Verification items for the finished model (mm, model axes). Coordinates: 2 decimals unless noted, no trailing zeros. Order: outer loops, then holes, each group sorted by start corner. A loop starts at its lowest first (then second) coordinate and runs counter-clockwise, first axis right, second up. Notation, with made-up numbers: (81.5, -21.5) -> (96.5, -21.5) arc R14 cw to (96.5, -1.5) -> close; hole circle Ø4 at (59, -12). An arc over 180 degrees is marked (long way). Use CSV: the item, a comma, the result in double quotes. Start each with the question number.
1) Release check for a two-part mould opening along X. For faces 1 (the flat face through (5.107, 38.792, 0.032)), 2 (the flat face through (-35, 10, 2.306)), 3 (the cylindrical face through (-42.5, 2.8, 0)) record: released by +X, released by -X, zero draft, split by the parting line, or undercut.
2) Go/stop test with flat-tipped pins: pin 1 (8 mm diameter, centred on x = -17, y = 21, fed in from +Z); pin 2 (1.5 mm diameter, centred on x = -25, z = -1.5, fed in from +Y). Record where each tip stops, or that it passes through.
3) Sectioned sample at A-A on y = 0. Record the boundary of the cut face in (x, z), then the cut area to 3 significant figures.
4) Sectioned sample at C-C on x = 0. Record the boundary of the cut face in (y, z).
5) Scan lines: line 1 along Y through (x, z) = (-8, 1.8); line 2 along Y through (x, z) = (2.5, -0.4); line 3 along Y through (x, z) = (-18, 0.5). Record each from-to range of solid material in increasing order.
6) Sectioned sample at B-B on z = 1.55. Give the number of separate pieces and of enclosed holes in the cut face, then the cut area to 3 significant figures.
from build123d import *

# Parameters (mm, degrees)
EXTRUDE5_DEPTH     = 2.30625
SKETCH31_R         = 0.396875
SKETCH31_R_2       = 1.0922
CUT_EXTRUDE4_DEPTH = 5.6125
CIRPATTERN1_COUNT  = 24
CIRPATTERN1_ANGLE  = 172.5
CUT_EXTRUDE5_DEPTH = 5.6125


with BuildPart() as part:
    # Sketch7 → Extrude5 (new body, symmetric)
    with BuildSketch(Plane.XY):
        with BuildLine():
            Line((5.87367865, 44.615018762), (4.568416728, 34.700570148))
            ThreePointArc((4.568416728, 34.700570148), (-34.700570148, 4.568416728), (-4.568416728, -34.700570148))
            Line((-4.568416728, -34.700570148), (-5.87367865, -44.615018762))
            ThreePointArc((-5.87367865, -44.615018762), (-44.615018762, 5.87367865), (5.87367865, 44.615018762))
        make_face()
    extrude(amount=EXTRUDE5_DEPTH, both=True)

    # Sketch31 → Cut-Extrude4 (cut, through all)
    with BuildSketch(Plane.XY.offset(2.30625)):
        with Locations((-7.315887076, -36.779448015)):
            Circle(SKETCH31_R)
        with Locations((-8.096248364, -40.702589137)):
            Circle(SKETCH31_R_2)
    cut_extrude4 = extrude(amount=-CUT_EXTRUDE4_DEPTH, mode=Mode.SUBTRACT)

    # CirPattern1: Cut-Extrude4 ×24 about axis
    cirpattern1_axis = Axis((0, 0, 0), (0, 0, -1))
    for i in range(1, CIRPATTERN1_COUNT):
        add(cut_extrude4.rotate(cirpattern1_axis, i * CIRPATTERN1_ANGLE / (CIRPATTERN1_COUNT - 1)), mode=Mode.SUBTRACT)

    # Sketch32 → Cut-Extrude5 (cut, through all)
    with BuildSketch(Plane.XY.offset(2.30625)):
        with BuildLine():
            Line((4.061625331, 44.816327378), (5.630931125, 42.77116825))
            Line((5.630931125, 42.77116825), (5.87367865, 44.615018762))
            ThreePointArc((5.87367865, 44.615018762), (4.968671612, 44.724851061), (4.061625331, 44.816327378))
        make_face()
    extrude(amount=-CUT_EXTRUDE5_DEPTH, mode=Mode.SUBTRACT)


solid = part.part
Answers follow:
1,face 1,"released by +X"
1,face 2,"zero draft"
1,face 3,"undercut"
2,pin 1,"passes through"
2,pin 2,"stops at y = 37.91"
3,outline,"(-45, -2.31) -> (-35, -2.31) -> (-35, 2.31) -> (-45, 2.31) -> close"
3,area,"46.1 mm²"
4,outline,"(35, -2.31) -> (45, -2.31) -> (45, 2.31) -> (35, 2.31) -> close"
5,line 1,"y = -44.28 to -41.79, -39.61 to -34.07, 34.07 to 39.61, 41.79 to 44.28"
5,line 2,"y = 34.91 to 37.03, 37.81 to 40.34, 42.48 to 44.93"
5,line 3,"y = -41.24 to -38.25, -36.19 to -30.02, 30.02 to 36.19, 38.25 to 41.24"
6,separate pieces,"1"
6,enclosed holes,"48"
6,area,"1,150 mm²"
